Could you check a few things on this drawing? It's one solid part, dimensions in mm from its lowest x, y, z. A direction names the side the tool comes from. Give positions to 0.01 mm unless a question says otherwise; leave off trailing zeros. Write each loop counter-clockwise with the first axis right and the second up, starting at its lowest first coordinate (ties: lowest second). Pieces come first, ordered by that corner, then holes. Notation, with made-up numbers: (23, -2.75) - (74, -2.75) arc R19 cw to (74, 18.25) - close; hole circle Ø3 at (-4.5, 42.25). An arc over 180 degrees is marked (long way). One line per item, written item: value. Start each with the question number.
1) Imagine slicing it at A-A on z = 20. Write out the boundary of the cut face in (x, y).
2) Please list where these lines run through material, in increasing order: L1, parallel to Y at x = 35, z = 30.5; L2, parallel to Z at x = 17, y = 11.25; L3, parallel to Z at x = 20, y = 8. Write a range as [from, to].
3) Imagine slicing it at C-C on y = 7.5. Write out the boundary of the cut face in (x, z).
4) Imagine slicing it at B-B on x = 20. Write out the boundary of the cut face in (y, z).
5) Imagine slicing it at D-D on x = 34. Write out the boundary of the cut face in (y, z).
6) I'm going to push flat-ended pins straight in: P1, Ø2, axis at x = 30.5, z = 18.5, coming from the +Y side; P2, Ø2, axis at x = 23.5, y = 8, coming from the -Z side. Where does each tip first touch, or does it pass through?
7) On a 3-axis mill with a long thin cutter (end or side, diameter ignored), from which of +Z, -Z, +X, -X, +Y, -Y can I reach the whole of each face in a straight line? I mean the marked faces 1 and 2. Say none if no direction works.
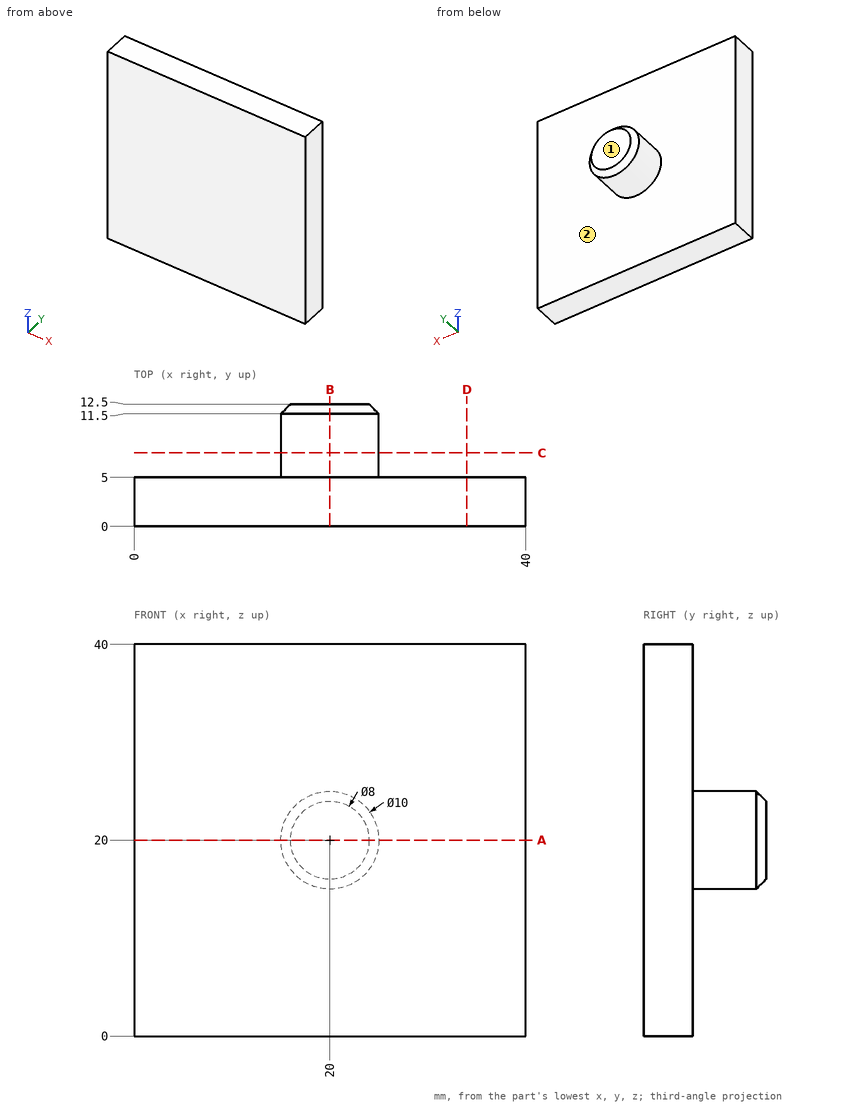
Numbers:
1. outline: (0, 0) - (40, 0) - (40, 5) - (25, 5) - (25, 11.5) - (24, 12.5) - (16, 12.5) - (15, 11.5) - (15, 5) - (0, 5) - close
2. L1: [0, 5]
2. L2: [16, 24]
2. L3: [15, 25]
3. outline: circle Ø10 at (20, 20)
4. outline: (0, 0) - (5, 0) - (5, 15) - (11.5, 15) - (12.5, 16) - (12.5, 24) - (11.5, 25) - (5, 25) - (5, 40) - (0, 40) - close
5. outline: (0, 0) - (5, 0) - (5, 40) - (0, 40) - close
6. P1: y = 5
6. P2: z = 15.67
7. face 1: +Z, -Z, +X, -X, +Y
7. face 2: +Y
